Could you check a few things on this model? Use its own coordinates, in mm. Coordinates: 2 decimals unless noted, no trailing zeros. Loops run counter-clockwise (first coordinate to the right, second up) from the corner with the lowest first, then second, coordinate; pieces in that order, holes last.
1) Imagine slicing it at A-A on z = 3.5. Give the number of separate pieces and of enclosed holes in the cut face, plus the area to 3 significant figures.
2) Imagine slicing it at D-D on y = 0. Please give me the cut outline in (x, z) (3 decimals).
3) If I drill on line 1 along X through (y, z) = (40.5, 3.25); line 2 along X through (y, z) = (36.5, 3); line 3 along Y through (x, z) = (0, 3.75) (3 decimals), over which ranges is the centre line in solid material (lowest first)?
4) Will these pins go through, and if not, where does the flat tip stop? P1, Ø6, axis at x = -42.5, y = 48.5, coming from the -Z side; P2, Ø3, axis at y = 46.5, z = 1.5, coming from the +X side; P3, Ø3, axis at y = 36.5, z = 2.5, coming from the -X side; P4, Ø3, axis at y = 42.5, z = 2.5, coming from the -X side.
5) Imagine slicing it at C-C on y = 44. Please give me the cut outline in (x, z), plus the area to 3 significant figures.
6) Imagine slicing it at B-B on x = 37.5. Please give me the cut outline in (y, z).
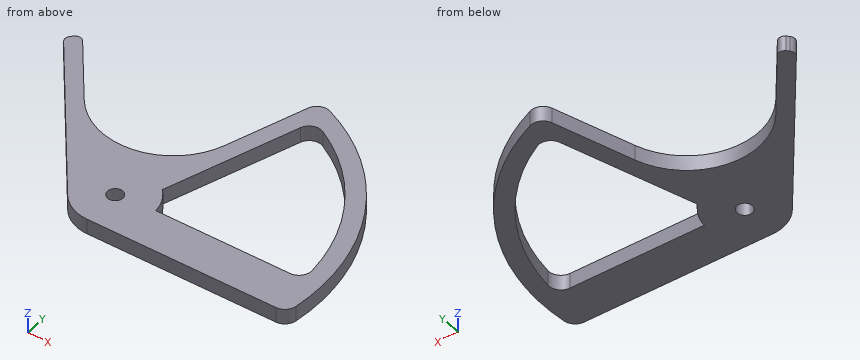
```python
from build123d import *

# Parameters (mm, degrees)
SKETCH1_R           = 3.175
BOSS_EXTRUDE1_DEPTH = 6.35
FILLET1_R           = 5.08
FILLET2_R           = 2.54


with BuildPart() as part:
    # Sketch1 → Boss-Extrude1 (new body)
    with BuildSketch(Plane.XY):
        with BuildLine():
            Line((-12.557727148, -9.711802813), (-62.907969157, 55.392958186))
            ThreePointArc((-62.907969157, 55.392958186), (-60.738998149, 57.76302021), (-58.480795155, 60.048222272))
            Line((-58.480795155, 60.048222272), (-37.93049883, 33.475914427))
            ThreePointArc((-37.93049883, 33.475914427), (-9.314173502, 22.341362046), (13.936413388, 42.398344403))
            Line((13.936413388, 42.398344403), (26.174060388, 79.628581318))
            ThreePointArc((26.174060388, 79.628581318), (72.040987894, 42.847269029), (82.4642609, -15.014595376))
            Line((82.4642609, -15.014595376), (0, -15.875))
            ThreePointArc((0, -15.875), (-6.994310379, -14.251148983), (-12.557727148, -9.711802813))
        make_face()
        Circle(SKETCH1_R, mode=Mode.SUBTRACT)
        with BuildLine():
            Line((30.398061223, 70.395411405), (11.01621883, 11.430596996))
            ThreePointArc((11.01621883, 11.430596996), (14.320406292, 6.851393189), (15.812676769, 1.405303663))
            Line((15.812676769, 1.405303663), (76.65111989, 2.04007171))
            ThreePointArc((76.65111989, 2.04007171), (63.505865166, 42.971632067), (30.398061223, 70.395411405))
        make_face(mode=Mode.SUBTRACT)
    extrude(amount=BOSS_EXTRUDE1_DEPTH)

    # Fillet1
    fillet1_edges = [part.edges().sort_by_distance(p)[0] for p in [
        (76.65111989, 2.04007171, 3.175),
        (30.398061223, 70.395411405, 3.175),
        (26.174060388, 79.628581318, 3.175),
        (82.4642609, -15.014595376, 3.175),
    ]]
    fillet(fillet1_edges, radius=FILLET1_R)

    # Fillet2
    fillet2_edges = [part.edges().sort_by_distance(p)[0] for p in [
        (-62.907969157, 55.392958186, 3.175),
        (-58.480795155, 60.048222272, 3.175),
    ]]
    fillet(fillet2_edges, radius=FILLET2_R)


solid = part.part
```
Filled in:
1. separate pieces: 1
1. enclosed holes: 2
1. area: 3,980 mm2
2. outline: (-20.069, 0) - (-3.175, 0) - (-3.175, 6.35) - (-20.069, 6.35) - close; (3.175, 0) - (83.82, 0) - (83.82, 6.35) - (3.175, 6.35) - close
3. line 1: x = -51.39 to -43.36, 13.24 to 20.57, 65.11 to 73.39
3. line 2: x = -48.3 to -40.27, 11.26 to 19.26, 67.43 to 75.46
3. line 3: y = -15.875 to -3.175, 3.175 to 25.602
4. P1: passes through
4. P2: stops at x = 70.72
4. P3: stops at x = -49.46
4. P4: stops at x = -54.1
5. outline: (-54.1, 0) - (-46.07, 0) - (-46.07, 6.35) - (-54.1, 6.35) - close; (14.46, 0) - (21.72, 0) - (21.72, 6.35) - (14.46, 6.35) - close; (62.8, 0) - (71.34, 0) - (71.34, 6.35) - (62.8, 6.35) - close
5. area: 151 mm2
6. outline: (-15.48, 0) - (1.63, 0) - (1.63, 6.35) - (-15.48, 6.35) - close; (66.88, 0) - (74.96, 0) - (74.96, 6.35) - (66.88, 6.35) - close
